Source: CAD feature listing. Evaluate the final solid. Frame: model axes, mm. A direction names the side the tool comes from. Coordinates: 2 decimals unless noted, no trailing zeros. Loops run counter-clockwise (first coordinate to the right, second up) from the corner with the lowest first, then second, coordinate; pieces in that order, holes last.
```python
from build123d import *

# Parameters (mm, degrees)
F1_W     = 22.3188386493
F1_H     = 30
F2_DEPTH = 50
F3_W     = 30
F3_H     = 25
F4_DEPTH = 30
F5_W     = 12.6015079648
F5_H     = 30
F6_DEPTH = 60
F7_W     = 90
F7_H     = 20
F8_DEPTH = 10


with BuildPart() as f2:
    # F1 (on Front) → F2 (new body)
    with BuildSketch(Plane.XZ):
        Polygon((20, 40), (20, 0), (110, 0), (110, 30), (63.4782647698, 30), (41.1594261205, 30), (41.1594261205, 60), (0, 60), (0, 40), align=None)
        with Locations((52.3188454451, 45)):
            Rectangle(F1_W, F1_H)
    extrude(amount=-F2_DEPTH)

    # F3 (on face) → F4 (cut)
    with BuildSketch(Plane.XY.offset(60)):
        with Locations((48.4782647698, 12.5)):
            Rectangle(F3_W, F3_H)
    extrude(amount=-F4_DEPTH, mode=Mode.SUBTRACT)

    # F5 (on face) → F6 (cut)
    with BuildSketch(Plane.XY.offset(60)):
        with Locations((6.3007539824, 25)):
            Rectangle(F5_W, F5_H)
    extrude(amount=-F6_DEPTH, mode=Mode.SUBTRACT)

    # F7 (on face) → F8 (cut)
    with BuildSketch(Plane(origin=(0, 0, 0), x_dir=(1, 0, 0), z_dir=(0, 0, -1))):
        with Locations((65, -25)):
            Rectangle(F7_W, F7_H)
    extrude(amount=-F8_DEPTH, mode=Mode.SUBTRACT)


solid = f2.part
```
Q1. Section query B-B on y = 23. Return the cut outline in (x, z).
Q2. Section query A-A on z = 8.5. Return the cut outline in (x, y), then the cut area to 3 significant figures.
Q3. Section query C-C on z = 41.5. Return the cut outline in (x, y).
Q4. Reachability of faces 4 (the flat face through (6, 40, 50)), 5 (the flat face through (64, 25, 10)), 6 (the flat face through (33.478, 12, 45)) from +Z, -Z, +X, -X, +Y, -Y: full face, straight path, thin tool, end or side. Return the list, or none.
Q5. First-contact query: pin 1 Ø12 at (y, z) = (24.5, 27) entering from -X; pin 2 Ø9 at (x, z) = (45, 51.5) entering from -Y; pin 3 Ø1 at (x, y) = (89, 14.5) entering from +Z; pin 4 Ø6 at (x, y) = (7, 25.5) entering from -Z. Flat tips, straight axial feed; report the tip coordinate or a pass-through.
Q6. Material intervals for line 1 along Y through (x, z) = (92, 6); line 2 along Z through (x, y) = (56, 24); line 3 along Z through (x, y) = (11, 40.5), sorted ascending.
Q7. Draft query along Y for faces 1 (the flat face through (20, 25, 20)), 2 (the flat face through (54, 0, 24)), 3 (the flat face through (64, 15, 5)). Return one class per face: released by +Y, released by -Y, zero draft, split by the parting line, or undercut.
Q8. Section query D-D on x = 35. Return the cut outline in (y, z).
Resolved:
1. outline: (12.6, 40) - (20, 40) - (20, 10) - (110, 10) - (110, 30) - (33.48, 30) - (33.48, 60) - (12.6, 60) - close
2. outline: (20, 0) - (110, 0) - (110, 15) - (20, 15) - close; (20, 35) - (110, 35) - (110, 50) - (20, 50) - close
2. area: 2,700 mm2
3. outline: (0, 0) - (33.48, 0) - (33.48, 25) - (63.48, 25) - (63.48, 50) - (0, 50) - (0, 40) - (12.6, 40) - (12.6, 10) - (0, 10) - close
4. face 4: +Z, -Z, -X
4. face 5: -Z, +X, -X
4. face 6: +Z, +X, -Y
5. pin 1: stops at x = 20
5. pin 2: stops at y = 25
5. pin 3: stops at z = 30
5. pin 4: passes through
6. line 1: y = 0 to 15, 35 to 50
6. line 2: z = 10 to 30
6. line 3: z = 40 to 60
7. face 1: zero draft
7. face 2: released by -Y
7. face 3: undercut
8. outline: (0, 0) - (15, 0) - (15, 10) - (35, 10) - (35, 0) - (50, 0) - (50, 60) - (25, 60) - (25, 30) - (0, 30) - close
